Design review of the part built by this model. Coordinates are the model's own, in mm. Face numbers are marked on the shaded views. A direction names the side the tool comes from. Round coordinates to 2 decimals unless told otherwise and drop trailing zeros. Order: outer loops, then holes, each group sorted by start corner. A loop starts at its lowest first (then second) coordinate and runs counter-clockwise, first axis right, second up. Notation, with made-up numbers: (68, 6) - (125, 6) arc R9 cw to (125, 17) - close; hole circle Ø3 at (39, 88). An arc over 180 degrees is marked (long way). Write item = value, one per line.
from build123d import *

# Parameters (mm, degrees)
SKETCH1_R               = 3.7625
PART1_DEPTH             = 14
SKETCH3_W               = 3
SKETCH3_H               = 4
KEYWAY1_DEPTH           = 13
SKETCH4_R               = 4.7625
PART2_BALLBEARING_DEPTH = 14
KEYWAY1_A_R             = 1.5
KEYWAY1_B_R             = 1.5
SKETCH6_R               = 6
PART3_DEPTH             = 5
SKETCH7_R               = 4.7625
PART4_DEPTH             = 13
SKETCH8_W               = 3
SKETCH8_H               = 4
KEYWAY2_DEPTH           = 13
SKETCH9_R               = 4.7625
PART5_BALLBEARING_DEPTH = 14
FILLET1_R               = 1.5
FILLET2_R               = 1.5


# Some blends are built 0.0001 mm under size
with BuildPart() as part:
    # Sketch1 → Part1 (new body)
    with BuildSketch(Plane.XY):
        Circle(SKETCH1_R)
    extrude(amount=PART1_DEPTH)

    # Sketch3 → Keyway1 (cut)
    with BuildSketch(Plane(origin=(0, 0, 0), x_dir=(-1, 0, 0), z_dir=(0, 0, -1))):
        with Locations((0, 3.7625)):
            Rectangle(SKETCH3_W, SKETCH3_H)
    extrude(amount=-KEYWAY1_DEPTH, mode=Mode.SUBTRACT)

    # Sketch4 → Part2_BallBearing (add)
    with BuildSketch(Plane(origin=(0, 0, 0), x_dir=(-1, 0, 0), z_dir=(0, 0, -1))):
        Circle(SKETCH4_R)
    extrude(amount=PART2_BALLBEARING_DEPTH)

    # Keyway1_a
    # the kernel refuses this fillet: 1.5 mm, written as the material it adds along each edge
    with BuildSketch(Plane(origin=(1.5, -1.9875, 0), x_dir=(-1, 0, 0), z_dir=(0, 1, 0))) as keyway1_a_piece_1_section:
        with BuildLine():
            CenterArc((KEYWAY1_A_R, KEYWAY1_A_R), KEYWAY1_A_R, 180, 90)
            Line((0, KEYWAY1_A_R), (0, 0))
            Line((0, 0), (KEYWAY1_A_R, 0))
        make_face()
    keyway1_a_piece_1 = extrude(amount=9.188066, mode=Mode.PRIVATE)
    keyway1_a_piece_1 = keyway1_a_piece_1 & Plane(origin=(0, 0, 0.327266), x_dir=(1, 0, 0), z_dir=(0, 0, -1)) * Cylinder(3.7625, 25, mode=Mode.PRIVATE)
    add(keyway1_a_piece_1)
    with BuildSketch(Plane(origin=(-1.5, 7.200566, 0), x_dir=(1, 0, 0), z_dir=(0, -1, 0))) as keyway1_a_piece_2_section:
        with BuildLine():
            CenterArc((KEYWAY1_A_R, KEYWAY1_A_R), KEYWAY1_A_R, 180, 90)
            Line((0, KEYWAY1_A_R), (0, 0))
            Line((0, 0), (KEYWAY1_A_R, 0))
        make_face()
    keyway1_a_piece_2 = extrude(amount=9.188066, mode=Mode.PRIVATE)
    keyway1_a_piece_2 = keyway1_a_piece_2 & Plane(origin=(0, 0, 0.327266), x_dir=(1, 0, 0), z_dir=(0, 0, -1)) * Cylinder(3.7625, 25, mode=Mode.PRIVATE)
    add(keyway1_a_piece_2)

    # Keyway1_b
    keyway1_b_edges = [part.edges().sort_by_distance(p)[0] for p in [
        (1.5, 2.606533, 13),
        (-1.5, 2.606533, 13),
    ]]
    fillet(keyway1_b_edges, radius=KEYWAY1_B_R - 0.0001)  # a hair under: the kernel refuses the full size

    # Sketch6 → Part3 (add)
    with BuildSketch(Plane(origin=(0, 0, -14), x_dir=(-1, 0, 0), z_dir=(0, 0, -1))):
        Circle(SKETCH6_R)
    extrude(amount=PART3_DEPTH)

    # Sketch7 → Part4 (add)
    with BuildSketch(Plane(origin=(0, 0, -19), x_dir=(-1, 0, 0), z_dir=(0, 0, -1))):
        Circle(SKETCH7_R)
    extrude(amount=PART4_DEPTH)

    # Sketch8 → KeyWay2 (cut)
    with BuildSketch(Plane(origin=(0, 0, -32), x_dir=(-1, 0, 0), z_dir=(0, 0, -1))):
        with Locations((0, 4.7625)):
            Rectangle(SKETCH8_W, SKETCH8_H)
    extrude(amount=-KEYWAY2_DEPTH, mode=Mode.SUBTRACT)

    # Sketch9 → Part5__BallBearing (add)
    with BuildSketch(Plane(origin=(0, 0, -32), x_dir=(-1, 0, 0), z_dir=(0, 0, -1))):
        Circle(SKETCH9_R)
    extrude(amount=PART5_BALLBEARING_DEPTH)

    # Fillet1
    # the kernel refuses this fillet: 1.5 mm, written as the material it adds along each edge
    with BuildSketch(Plane(origin=(1.5, -0.9875, -19), x_dir=(-1, 0, 0), z_dir=(0, 1, 0))) as fillet1_piece_1_section:
        with BuildLine():
            CenterArc((FILLET1_R, -FILLET1_R), FILLET1_R, 90, 90)
            Line((0, -FILLET1_R), (0, 0))
            Line((0, 0), (FILLET1_R, 0))
        make_face()
    fillet1_piece_1 = extrude(amount=9.257611, mode=Mode.PRIVATE)
    fillet1_piece_1 = fillet1_piece_1 & Plane(origin=(0, 0, -19.329162), x_dir=(-1, 0, 0), z_dir=(0, 0, 1)) * Cylinder(4.7625, 25, mode=Mode.PRIVATE)
    add(fillet1_piece_1)
    with BuildSketch(Plane(origin=(-1.5, 8.270111, -19), x_dir=(1, 0, 0), z_dir=(0, -1, 0))) as fillet1_piece_2_section:
        with BuildLine():
            CenterArc((FILLET1_R, -FILLET1_R), FILLET1_R, 90, 90)
            Line((0, -FILLET1_R), (0, 0))
            Line((0, 0), (FILLET1_R, 0))
        make_face()
    fillet1_piece_2 = extrude(amount=9.257611, mode=Mode.PRIVATE)
    fillet1_piece_2 = fillet1_piece_2 & Plane(origin=(0, 0, -19.329163), x_dir=(-1, 0, 0), z_dir=(0, 0, 1)) * Cylinder(4.7625, 25, mode=Mode.PRIVATE)
    add(fillet1_piece_2)

    # Fillet2
    # the kernel refuses this fillet: 1.5 mm, written as the material it adds along each edge
    with BuildSketch(Plane(origin=(1.5, -0.9875, -32), x_dir=(-1, 0, 0), z_dir=(0, 1, 0))) as fillet2_piece_1_section:
        with BuildLine():
            CenterArc((FILLET2_R, FILLET2_R), FILLET2_R, 180, 90)
            Line((0, FILLET2_R), (0, 0))
            Line((0, 0), (FILLET2_R, 0))
        make_face()
    fillet2_piece_1 = extrude(amount=9.257611, mode=Mode.PRIVATE)
    fillet2_piece_1 = fillet2_piece_1 & Plane(origin=(0, 0, -31.660407), x_dir=(-1, 0, 0), z_dir=(0, 0, 1)) * Cylinder(4.7625, 25, mode=Mode.PRIVATE)
    add(fillet2_piece_1)
    with BuildSketch(Plane(origin=(-1.5, 8.270111, -32), x_dir=(0, 0, 1), z_dir=(0, -1, 0))) as fillet2_piece_2_section:
        with BuildLine():
            CenterArc((FILLET2_R, -FILLET2_R), FILLET2_R, 90, 90)
            Line((0, -FILLET2_R), (0, 0))
            Line((0, 0), (FILLET2_R, 0))
        make_face()
    fillet2_piece_2 = extrude(amount=9.257611, mode=Mode.PRIVATE)
    fillet2_piece_2 = fillet2_piece_2 & Plane(origin=(0, 0, -31.668087), x_dir=(-1, 0, 0), z_dir=(0, 0, 1)) * Cylinder(4.7625, 25, mode=Mode.PRIVATE)
    add(fillet2_piece_2)


solid = part.part
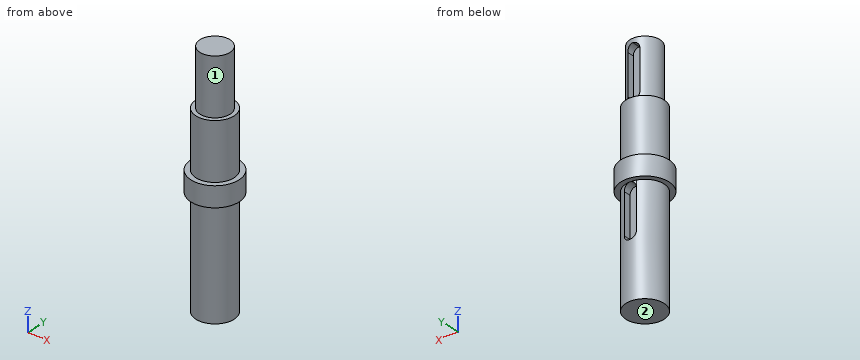
1) For the marked faces 1 and 2, list the 3-axis set-ups (+Z, -Z, +X, -X, +Y, -Y) from which the entire face can be reached by the end or side of a thin tool; tool diameter is ignored.
Findings:
face_1 = +Z
face_2 = -Z, +X, -X, +Y, -Y
2) We need section B-B on z = 5. Write out the cut boundary in (x, y) (1 decimal), and give its area (3 significant figures).
Findings:
outline = (-1.5, 1.8) - (-1.5, 3.5) arc R3.8 ccw (long way) to (1.5, 3.5) - (1.5, 1.8) - close
area = 38.8 mm^2
3) We need section C-C on x = 1. Write out the cut boundary in (y, z), and give its area (3 significant figures).
Findings:
outline = (-5.92, -19) - (-4.66, -19) - (-4.66, -46) - (4.66, -46) - (4.66, -31.62) - (2.76, -31.62) - (2.76, -19.38) - (4.66, -19.38) - (4.66, -19) - (5.92, -19) - (5.92, -14) - (4.66, -14) - (4.66, 0) - (3.63, 0) - (3.63, 0.38) - (1.76, 0.38) - (1.76, 12.62) - (3.63, 12.62) - (3.63, 14) - (-3.63, 14) - (-3.63, 0) - (-4.66, 0) - (-4.66, -14) - (-5.92, -14) - close
area = 497 mm^2
4) To check wall thickness, follow L1, parallel to Y at x = 0.25, z = -18; L2, parallel to Z at x = -5.5, y = 0.75; L3, parallel to Z at x = 4, y = 2.25. State the ranges of each line that lie inside material, in increasing order. Write a range as from..to.
Findings:
L1 = -5.99..5.99
L2 = -19..-14
L3 = -46..0
5) We need section D-D on z = -31. Write out the cut boundary in (x, y) (1 decimal).
Findings:
outline = (-1.4, 2.8) - (-1.4, 4.5) arc R4.8 ccw (long way) to (1.4, 4.5) - (1.4, 2.8) - close
6) Clearance check with flat-ended pins moving along their axes: pin 1 Ø1.9 at (y, z) = (3.5, -23) entering from +X; pin 2 Ø4 at (y, z) = (1.5, -39.5) entering from -X; pin 3 Ø1.5 at (y, z) = (-2.5, -25) entering from -X. State where each tip first meets the part, or that it passes through.
Findings:
pin_1 = 4.02
pin_2 = -4.76
pin_3 = -4.43
7) We need section A-A on y = -1. Write out the cut boundary in (x, z).
Findings:
outline = (-5.92, -19) - (-4.66, -19) - (-4.66, -46) - (4.66, -46) - (4.66, -19) - (5.92, -19) - (5.92, -14) - (4.66, -14) - (4.66, 0) - (3.63, 0) - (3.63, 14) - (-3.63, 14) - (-3.63, 0) - (-4.66, 0) - (-4.66, -14) - (-5.92, -14) - close
